from build123d import *

# Parameters (mm, degrees)
UPPER_BOLT_HOLES_REACH  = 90.9
SKETCH4_R               = 2.0193
SKETCH6_R               = 2.0193
LOWER_BOLT_HOLES_DEPTH  = 12.7
SKETCH7_W               = 56.79526179
SKETCH7_H               = 3.81
SKETCH8_W               = 48.26
SKETCH8_H               = 19.05
SIDEWALL_CUTOUT_1_DEPTH = 76.2
SKETCH10_W              = 48.26
SKETCH10_H              = 19.05
SIDEWALL_CUTOUT_2_DEPTH = 76.2
SKETCH11_W              = 50.8
SKETCH11_H              = 19.05
SIDEWALL_CUTOUT_3_DEPTH = 76.2
SKETCH13_W              = 48.26
SKETCH13_H              = 19.05
SIDEWALL_CUTOUT_4_DEPTH = 76.2


with BuildPart() as part:
    # Sketch1 → Revolve1 (revolve)
    with BuildSketch(Plane.XY):
        Polygon((-88.9, 54.61), (-88.9, 44.45), (0, 44.45), (0, 63.5), (-25.4, 63.5), (-25.4, 54.61), align=None)
    revolve(axis=Axis((-87.283636364, 0, 0), (1, 0, 0)))

    # Sketch4 → Upper Bolt Holes (cut, up to next)
    with BuildSketch(Plane(origin=(0, 0, 0), x_dir=(0, 0, -1), z_dir=(1, 0, 0)), mode=Mode.PRIVATE) as upper_bolt_holes_sk1:
        with Locations((56.020377392, 16.571472984)):
            Circle(SKETCH4_R)
    upper_bolt_holes_tool1 = extrude(upper_bolt_holes_sk1.sketch, amount=-UPPER_BOLT_HOLES_REACH, mode=Mode.PRIVATE) & part.part
    add(upper_bolt_holes_tool1.solids().sort_by_distance((0, 16.571473, -56.020377))[0], mode=Mode.SUBTRACT)
    # Sketch4 → Upper Bolt Holes (cut, up to next)
    with BuildSketch(Plane(origin=(0, 0, 0), x_dir=(0, 0, -1), z_dir=(1, 0, 0)), mode=Mode.PRIVATE) as upper_bolt_holes_sk2:
        with Locations((56.800806443, -13.658872113)):
            Circle(SKETCH4_R)
    upper_bolt_holes_tool2 = extrude(upper_bolt_holes_sk2.sketch, amount=-UPPER_BOLT_HOLES_REACH, mode=Mode.PRIVATE) & part.part
    add(upper_bolt_holes_tool2.solids().sort_by_distance((0, -13.658872, -56.800806))[0], mode=Mode.SUBTRACT)
    # Sketch4 → Upper Bolt Holes (cut, up to next)
    with BuildSketch(Plane(origin=(0, 0, 0), x_dir=(0, 0, -1), z_dir=(1, 0, 0)), mode=Mode.PRIVATE) as upper_bolt_holes_sk3:
        with Locations((42.361505278, -40.229333459)):
            Circle(SKETCH4_R)
    upper_bolt_holes_tool3 = extrude(upper_bolt_holes_sk3.sketch, amount=-UPPER_BOLT_HOLES_REACH, mode=Mode.PRIVATE) & part.part
    add(upper_bolt_holes_tool3.solids().sort_by_distance((0, -40.229333, -42.361505))[0], mode=Mode.SUBTRACT)
    # Sketch4 → Upper Bolt Holes (cut, up to next)
    with BuildSketch(Plane(origin=(0, 0, 0), x_dir=(0, 0, -1), z_dir=(1, 0, 0)), mode=Mode.PRIVATE) as upper_bolt_holes_sk4:
        with Locations((16.571472984, -56.020377392)):
            Circle(SKETCH4_R)
    upper_bolt_holes_tool4 = extrude(upper_bolt_holes_sk4.sketch, amount=-UPPER_BOLT_HOLES_REACH, mode=Mode.PRIVATE) & part.part
    add(upper_bolt_holes_tool4.solids().sort_by_distance((0, -56.020377, -16.571473))[0], mode=Mode.SUBTRACT)
    # Sketch4 → Upper Bolt Holes (cut, up to next)
    with BuildSketch(Plane(origin=(0, 0, 0), x_dir=(0, 0, -1), z_dir=(1, 0, 0)), mode=Mode.PRIVATE) as upper_bolt_holes_sk5:
        with Locations((-13.658872113, -56.800806443)):
            Circle(SKETCH4_R)
    upper_bolt_holes_tool5 = extrude(upper_bolt_holes_sk5.sketch, amount=-UPPER_BOLT_HOLES_REACH, mode=Mode.PRIVATE) & part.part
    add(upper_bolt_holes_tool5.solids().sort_by_distance((0, -56.800806, 13.658872))[0], mode=Mode.SUBTRACT)
    # Sketch4 → Upper Bolt Holes (cut, up to next)
    with BuildSketch(Plane(origin=(0, 0, 0), x_dir=(0, 0, -1), z_dir=(1, 0, 0)), mode=Mode.PRIVATE) as upper_bolt_holes_sk6:
        with Locations((-40.229333459, -42.361505278)):
            Circle(SKETCH4_R)
    upper_bolt_holes_tool6 = extrude(upper_bolt_holes_sk6.sketch, amount=-UPPER_BOLT_HOLES_REACH, mode=Mode.PRIVATE) & part.part
    add(upper_bolt_holes_tool6.solids().sort_by_distance((0, -42.361505, 40.229333))[0], mode=Mode.SUBTRACT)
    # Sketch4 → Upper Bolt Holes (cut, up to next)
    with BuildSketch(Plane(origin=(0, 0, 0), x_dir=(0, 0, -1), z_dir=(1, 0, 0)), mode=Mode.PRIVATE) as upper_bolt_holes_sk7:
        with Locations((-56.020377392, -16.571472984)):
            Circle(SKETCH4_R)
    upper_bolt_holes_tool7 = extrude(upper_bolt_holes_sk7.sketch, amount=-UPPER_BOLT_HOLES_REACH, mode=Mode.PRIVATE) & part.part
    add(upper_bolt_holes_tool7.solids().sort_by_distance((0, -16.571473, 56.020377))[0], mode=Mode.SUBTRACT)
    # Sketch4 → Upper Bolt Holes (cut, up to next)
    with BuildSketch(Plane(origin=(0, 0, 0), x_dir=(0, 0, -1), z_dir=(1, 0, 0)), mode=Mode.PRIVATE) as upper_bolt_holes_sk8:
        with Locations((-56.800806443, 13.658872113)):
            Circle(SKETCH4_R)
    upper_bolt_holes_tool8 = extrude(upper_bolt_holes_sk8.sketch, amount=-UPPER_BOLT_HOLES_REACH, mode=Mode.PRIVATE) & part.part
    add(upper_bolt_holes_tool8.solids().sort_by_distance((0, 13.658872, 56.800806))[0], mode=Mode.SUBTRACT)
    # Sketch4 → Upper Bolt Holes (cut, up to next)
    with BuildSketch(Plane(origin=(0, 0, 0), x_dir=(0, 0, -1), z_dir=(1, 0, 0)), mode=Mode.PRIVATE) as upper_bolt_holes_sk9:
        with Locations((40.229333459, 42.361505278)):
            Circle(SKETCH4_R)
    upper_bolt_holes_tool9 = extrude(upper_bolt_holes_sk9.sketch, amount=-UPPER_BOLT_HOLES_REACH, mode=Mode.PRIVATE) & part.part
    add(upper_bolt_holes_tool9.solids().sort_by_distance((0, 42.361505, -40.229333))[0], mode=Mode.SUBTRACT)
    # Sketch4 → Upper Bolt Holes (cut, up to next)
    with BuildSketch(Plane(origin=(0, 0, 0), x_dir=(0, 0, -1), z_dir=(1, 0, 0)), mode=Mode.PRIVATE) as upper_bolt_holes_sk10:
        with Locations((13.658872113, 56.800806443)):
            Circle(SKETCH4_R)
    upper_bolt_holes_tool10 = extrude(upper_bolt_holes_sk10.sketch, amount=-UPPER_BOLT_HOLES_REACH, mode=Mode.PRIVATE) & part.part
    add(upper_bolt_holes_tool10.solids().sort_by_distance((0, 56.800806, -13.658872))[0], mode=Mode.SUBTRACT)
    # Sketch4 → Upper Bolt Holes (cut, up to next)
    with BuildSketch(Plane(origin=(0, 0, 0), x_dir=(0, 0, -1), z_dir=(1, 0, 0)), mode=Mode.PRIVATE) as upper_bolt_holes_sk11:
        with Locations((-16.571472984, 56.020377392)):
            Circle(SKETCH4_R)
    upper_bolt_holes_tool11 = extrude(upper_bolt_holes_sk11.sketch, amount=-UPPER_BOLT_HOLES_REACH, mode=Mode.PRIVATE) & part.part
    add(upper_bolt_holes_tool11.solids().sort_by_distance((0, 56.020377, 16.571473))[0], mode=Mode.SUBTRACT)
    # Sketch4 → Upper Bolt Holes (cut, up to next)
    with BuildSketch(Plane(origin=(0, 0, 0), x_dir=(0, 0, -1), z_dir=(1, 0, 0)), mode=Mode.PRIVATE) as upper_bolt_holes_sk12:
        with Locations((-42.361505278, 40.229333459)):
            Circle(SKETCH4_R)
    upper_bolt_holes_tool12 = extrude(upper_bolt_holes_sk12.sketch, amount=-UPPER_BOLT_HOLES_REACH, mode=Mode.PRIVATE) & part.part
    add(upper_bolt_holes_tool12.solids().sort_by_distance((0, 40.229333, 42.361505))[0], mode=Mode.SUBTRACT)

    # Sketch6 → Lower Bolt Holes (cut)
    with BuildSketch(Plane.ZY.offset(88.9)):
        with Locations((-10.905164891, 48.314576255)):
            Circle(SKETCH6_R)
        with Locations((26.452448456, 41.874680544)):
            Circle(SKETCH6_R)
        with Locations((48.314576255, 10.905164891)):
            Circle(SKETCH6_R)
        with Locations((41.874680544, -26.452448456)):
            Circle(SKETCH6_R)
        with Locations((10.905164891, -48.314576255)):
            Circle(SKETCH6_R)
        with Locations((-26.452448456, -41.874680544)):
            Circle(SKETCH6_R)
        with Locations((-48.314576255, -10.905164891)):
            Circle(SKETCH6_R)
        with Locations((-41.874680544, 26.452448456)):
            Circle(SKETCH6_R)
    extrude(amount=-LOWER_BOLT_HOLES_DEPTH, mode=Mode.SUBTRACT)

    # Sketch7 → 0.15in Depth Air Gap (revolve, cut)
    with BuildSketch(Plane.XY):
        with Locations((-46.425488876, 46.355)):
            Rectangle(SKETCH7_W, SKETCH7_H)
    revolve(axis=Axis((-102.668560336, 0, 0), (1, 0, 0)), mode=Mode.SUBTRACT)

    # Sketch8 → SideWall Cutout 1 (cut, symmetric)
    with BuildSketch(Plane(origin=(0, 0, 0), x_dir=(1, 0, 0), z_dir=(0, 1, 0))):
        with Locations((-50.8, 0)):
            Rectangle(SKETCH8_W, SKETCH8_H)
    extrude(amount=SIDEWALL_CUTOUT_1_DEPTH, both=True, mode=Mode.SUBTRACT)

    # Sketch10 → SideWall Cutout 2 (cut, symmetric)
    with BuildSketch(Plane.XY):
        with Locations((-50.8, 0)):
            Rectangle(SKETCH10_W, SKETCH10_H)
    extrude(amount=SIDEWALL_CUTOUT_2_DEPTH, both=True, mode=Mode.SUBTRACT)

    # Sketch11 → SideWall Cutout 3 (cut, symmetric)
    with BuildSketch(Plane(origin=(0, 0, 0), x_dir=(-1, 0, 0), z_dir=(0, 0.707106781, 0.707106781))):
        with Locations((50.8, 0)):
            Rectangle(SKETCH11_W, SKETCH11_H)
    extrude(amount=SIDEWALL_CUTOUT_3_DEPTH, both=True, mode=Mode.SUBTRACT)

    # Sketch13 → SideWall Cutout 4 (cut, symmetric)
    with BuildSketch(Plane(origin=(0, 0, 0), x_dir=(-1, 0, 0), z_dir=(0, -0.707106781, 0.707106781))):
        with Locations((50.8, 0)):
            Rectangle(SKETCH13_W, SKETCH13_H)
    extrude(amount=SIDEWALL_CUTOUT_4_DEPTH, both=True, mode=Mode.SUBTRACT)


solid = part.part
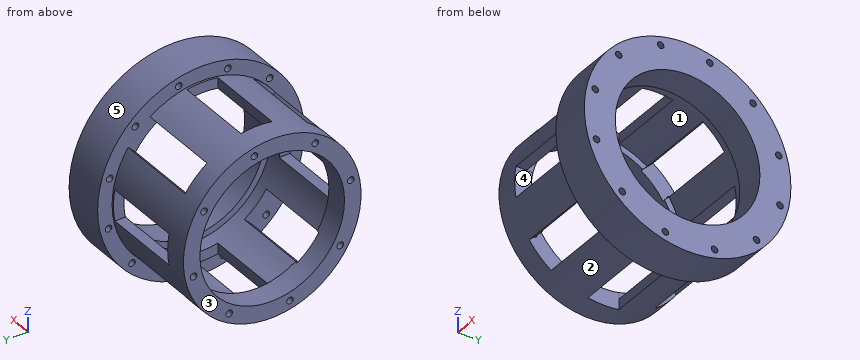
The model under review builds one solid part; all positions refer to its coordinate system, in mm. Face numbers are marked on the shaded views. A direction names the side the tool comes from. Give positions to 0.01 mm unless a question says otherwise; leave off trailing zeros. Write each loop counter-clockwise with the first axis right and the second up, starting at its lowest first coordinate (ties: lowest second). Pieces come first, ordered by that corner, then holes. Notation, with made-up numbers: M 56.5,-16.5 L 73.5,-16.5 A31 ccw 73.5,21.5 Z; hole C -8.5,-10.75 d2. An arc over 180 degrees is marked long. One line per question, with ' | ' between items. Start each with the question number.
Item 1: We need section C-C on x = -5. Give the number of separate pieces and of enclosed holes in the cut face, plus the area to 3 significant figures.
Item 2: We need section A-A on y = 0. Write out the cut boundary in (x, z).
Item 3: Draft analysis for pull direction Z (two halves, no side actions). For the marked faces 1, 2 and 3, state which applies: released by +Z, released by -Z, zero draft, split by the parting line, or undercut.
Item 4: For pin 1 (5 mm diameter, centred on y = 40.5, z = -15.5, fed in from +X); pin 2 (4 mm diameter, centred on y = 46, z = 35, fed in from -X); pin 3 (5 mm diameter, centred on x = -20, y = 45.5, fed in from +Z); pin 4 (11.5 mm diameter, centred on x = -62.5, y = -51, fed in from +Z), all flat-tipped, find the tip position at first contact; note any pin that passes through.
Item 5: Wall thickness on line 1 (Y direction, x = -18.5, z = -16); line 2 (X direction, y = -42, z = -17.5); line 3 (Y direction, x = -81, z = 10): over which ranges is each line inside the solid? List them lowest first. Write a range as from..to.
Item 6: For the marked faces 4 and 5, list the 3-axis set-ups (+Z, -Z, +X, -X, +Y, -Y) from which the entire face can be reached by the end or side of a thin tool; tool diameter is ignored.
Results found:
1) separate pieces: 1 | enclosed holes: 13 | area: 6,310 mm2
2) outline: M -88.9,-54.61 L -74.93,-54.61 L -74.93,-44.45 L -88.9,-44.45 Z; M -88.9,44.45 L -74.93,44.45 L -74.93,54.61 L -88.9,54.61 Z; M -26.67,-54.61 L -25.4,-54.61 L -25.4,-63.5 L 0,-63.5 L 0,-44.45 L -18.03,-44.45 L -18.03,-48.26 L -26.67,-48.26 Z; M -26.67,48.26 L -18.03,48.26 L -18.03,44.45 L 0,44.45 L 0,63.5 L -25.4,63.5 L -25.4,54.61 L -26.67,54.61 Z
3) face 1: undercut | face 2: split by the parting line | face 3: zero draft
4) pin 1: stops at x = 0 | pin 2: stops at x = -25.4 | pin 3: stops at z = 46.73 | pin 4: stops at z = 30.57
5) line 1: y = -61.45..-57.96, -54.08..-45.53, 45.53..61.45 | line 2: x = -88.9..-74.82, -18.03..0 | line 3: y = -53.69..-50.12, -46.51..-43.31, 43.31..53.69
6) face 4: +Y, -Y | face 5: +X, -X
